Here's the drawing with two shaded views (mm, measured from the low corner). I have some questions. A direction names the side the tool comes from. Round coordinates to 2 decimals unless told otherwise and drop trailing zeros. Loops run counter-clockwise (first coordinate to the right, second up) from the corner with the lowest first, then second, coordinate; pieces in that order, holes last.
(1) I want a section at C-C on x = 30. Write out the boundary of the cut face in (y, z).
(2) Will this pin go through, and if not, where does the flat tip stop? pin 1 Ø4 at (x, z) = (33.5, 41.5) entering from +Y.
(3) I want a section at D-D on y = 18. Write out the boundary of the cut face in (x, z), plus the area to 3 significant figures.
(4) If I drill on line 1 along X through (y, z) = (9.2, 30); line 2 along Z through (x, y) = (31, 25.5), over which ranges is the centre line in solid material (lowest first)?
(5) Thinking about a two-plate mould opening in Z: for the marked faces 1, 2 and 3, which applies, released by +Z, released by -Z, zero draft, split by the parting line, or undercut?
(6) I want a section at A-A on y = 23.25. Write out the boundary of the cut face in (x, z), plus the area to 3 significant figures.
(7) Which directions (+Z, -Z, +X, -X, +Y, -Y) give clear straight access to the entire face, cutting with the end or side of a thin tool? Please do the marked faces 4 and 5.
(8) I want a section at B-B on z = 30. Write out the boundary of the cut face in (x, y), plus the area to 3 significant figures.
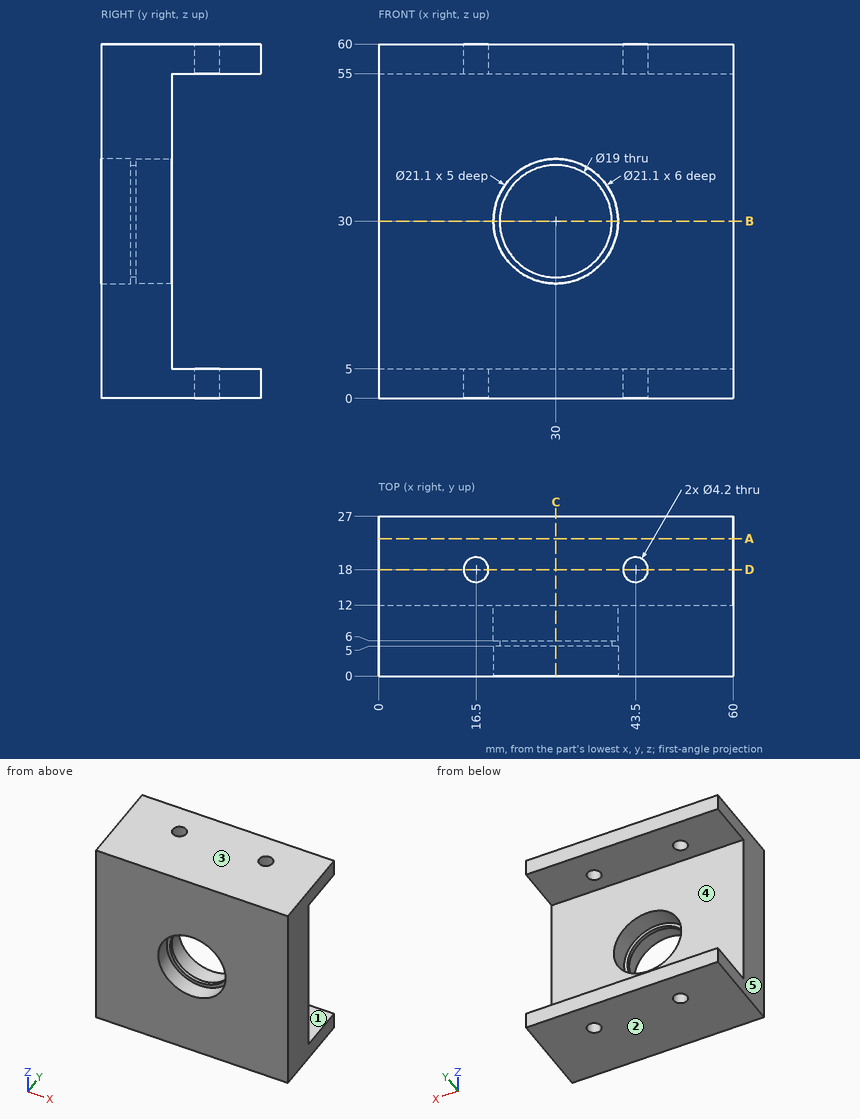
Filled sheet:
1. outline: (0, 0) - (27, 0) - (27, 5) - (12, 5) - (12, 19.45) - (6, 19.45) - (6, 20.5) - (5, 20.5) - (5, 19.45) - (0, 19.45) - close; (0, 40.55) - (5, 40.55) - (5, 39.5) - (6, 39.5) - (6, 40.55) - (12, 40.55) - (12, 55) - (27, 55) - (27, 60) - (0, 60) - close
2. pin 1: stops at y = 12
3. outline: (0, 0) - (14.4, 0) - (14.4, 5) - (0, 5) - close; (0, 55) - (14.4, 55) - (14.4, 60) - (0, 60) - close; (18.6, 0) - (41.4, 0) - (41.4, 5) - (18.6, 5) - close; (18.6, 55) - (41.4, 55) - (41.4, 60) - (18.6, 60) - close; (45.6, 0) - (60, 0) - (60, 5) - (45.6, 5) - close; (45.6, 55) - (60, 55) - (60, 60) - (45.6, 60) - close
3. area: 516 mm2
4. line 1: x = 0 to 19.45, 40.55 to 60
4. line 2: z = 0 to 5, 55 to 60
5. face 1: undercut
5. face 2: released by -Z
5. face 3: released by +Z
6. outline: (0, 0) - (60, 0) - (60, 5) - (0, 5) - close; (0, 55) - (60, 55) - (60, 60) - (0, 60) - close
6. area: 600 mm2
7. face 4: +X, -X, +Y
7. face 5: +Z, -Z, -X, +Y, -Y
8. outline: (0, 0) - (19.45, 0) - (19.45, 5) - (20.5, 5) - (20.5, 6) - (19.45, 6) - (19.45, 12) - (0, 12) - close; (39.5, 5) - (40.55, 5) - (40.55, 0) - (60, 0) - (60, 12) - (40.55, 12) - (40.55, 6) - (39.5, 6) - close
8. area: 469 mm2
